```python
from build123d import *

# Parameters (mm, degrees)
ESTRUSIONE_ESTRUSIONE1_DEPTH = 5
SCHIZZO2_R                   = 1.625
TAGLIO_ESTRUSIONE1_DEPTH     = 10.274243706
SCHIZZO3_R                   = 2.5
TAGLIO_ESTRUSIONE2_DEPTH     = 3.5


with BuildPart() as part:
    # Schizzo1 → Estrusione-Estrusione1 (new body, symmetric)
    with BuildSketch(Plane(origin=(0, 0, 0), x_dir=(0, 0, -1), z_dir=(1, 0, 0))):
        Polygon((-21.188457268, 88.94490566), (-26.688457268, 88.94490566), (-26.688457268, 109.666731067), (-40, 122.978273799), (-40, 156.723080253), (-25, 171.723080253), (-25, 168.94490566), (-22.828427125, 168.94490566), (-18.828427125, 172.94490566), (-17.414213562, 171.530692098), (-34.5, 154.44490566), (-34.5, 125.256448392), (-21.188457268, 111.94490566), align=None)
    extrude(amount=ESTRUSIONE_ESTRUSIONE1_DEPTH, both=True)

    # Schizzo2 → Taglio-Estrusione1 (cut, through all)
    with BuildSketch(Plane.XY.offset(26.688457268)):
        with Locations((0, 92.723474812)):
            Circle(SCHIZZO2_R)
    extrude(amount=-TAGLIO_ESTRUSIONE1_DEPTH, mode=Mode.SUBTRACT)

    # Schizzo3 → Taglio-Estrusione2 (cut)
    with BuildSketch(Plane.XY.offset(26.688457268)):
        with Locations((0, 92.723474812)):
            Circle(SCHIZZO3_R)
    extrude(amount=-TAGLIO_ESTRUSIONE2_DEPTH, mode=Mode.SUBTRACT)


solid = part.part
```
Work out the finished part from the listing and answer in its coordinate system (mm). A direction names the side the tool comes from. Coordinates: 2 decimals unless noted, no trailing zeros. Loops run counter-clockwise (first coordinate to the right, second up) from the corner with the lowest first, then second, coordinate; pieces in that order, holes last. Notation, with made-up numbers: (16.25, -35) - (23.25, -35) arc R15 cw to (23.25, -17) - close; hole circle Ø8 at (39.5, 43). An arc over 180 degrees is marked (long way). Use a Markdown table: item, result.
Item 1: For faces 4 (the cylindrical face through (-0.33, 95.2, 24.96)), 5 (the flat face through (0.07, 118.694, 27.937)), 6 (the flat face through (0, 99, 26.688)), 7 (the flat face through (0, 170, 25)), 8 (the flat face through (0, 101, 21.188)), determine the directions among +Z, -Z, +X, -X, +Y, -Y from which every point of the face is accessible in a straight line to the end or side of a thin tool.
Evaluation:
| item | result |
|---|---|
| face 4 | +Z |
| face 5 | -Z, +X, -X |
| face 6 | +Z, +X, -X, -Y |
| face 7 | +X, -X, +Y |
| face 8 | -Z, +X, -X, -Y |
Item 2: Find section A-A, the plane x = 0. Determine the outline of the cut face in (y, z), and give its area (3 significant figures).
Evaluation:
| item | result |
|---|---|
| outline | (88.94, 21.19) - (91.1, 21.19) - (91.1, 23.19) - (90.22, 23.19) - (90.22, 26.69) - (88.94, 26.69) - close; (94.35, 21.19) - (111.94, 21.19) - (125.26, 34.5) - (154.44, 34.5) - (171.53, 17.41) - (172.94, 18.83) - (168.94, 22.83) - (168.94, 25) - (171.72, 25) - (156.72, 40) - (122.98, 40) - (109.67, 26.69) - (95.22, 26.69) - (95.22, 23.19) - (94.35, 23.19) - close |
| area | 490 mm2 |
Item 3: Find section D-D, the plane y = 103. Determine the outline of the cut face in (x, z).
Evaluation:
| item | result |
|---|---|
| outline | (-5, 21.19) - (5, 21.19) - (5, 26.69) - (-5, 26.69) - close |
Item 4: The mould has two halves that part along Z. Classify faces 1 (the flat face through (0, 140, 34.5)), 2 (the flat face through (0.07, 170.917, 20.856)), 3 (the cylindrical face through (0.75, 91.28, 22.2)): +Z half, -Z half, draft (parallel to the pull), parting line (faces both ways), or undercut.
Evaluation:
| item | result |
|---|---|
| face 1 | -Z half |
| face 2 | undercut |
| face 3 | draft |
Item 5: Find section B-B, the plane z = 30.25. Determine the outline of the cut face in (x, y).
Evaluation:
| item | result |
|---|---|
| outline | (-5, 113.23) - (5, 113.23) - (5, 121.01) - (-5, 121.01) - close; (-5, 158.69) - (5, 158.69) - (5, 166.47) - (-5, 166.47) - close |
Item 6: Find section C-C, the plane x = -3.5. Determine the outline of the cut face in (y, z), and give its area (3 significant figures).
Evaluation:
| item | result |
|---|---|
| outline | (88.94, 21.19) - (111.94, 21.19) - (125.26, 34.5) - (154.44, 34.5) - (171.53, 17.41) - (172.94, 18.83) - (168.94, 22.83) - (168.94, 25) - (171.72, 25) - (156.72, 40) - (122.98, 40) - (109.67, 26.69) - (88.94, 26.69) - close |
| area | 514 mm2 |
Item 7: Given pin 1 Ø5 at (x, y) = (2, 138.5) entering from -Z; pin 2 Ø4 at (x, z) = (1.5, 28) entering from +Y; pin 3 Ø1.1 at (x, z) = (0, 23.5) entering from +Y; pin 4 Ø1.9 at (x, y) = (0, 92.72) entering from +Z, each flat-ended and moving along its own axis, determine where each tip first touches the part or whether it passes through.
Evaluation:
| item | result |
|---|---|
| pin 1 | stops at z = 34.5 |
| pin 2 | stops at y = 170.72 |
| pin 3 | stops at y = 168.94 |
| pin 4 | passes through |
Item 8: Consider probe 1 along Y at (x, z) = (0, 22.25); probe 2 along Y at (x, z) = (0, 22.7); probe 3 along Z at (x, y) = (-3.25, 154). Determine where each line is inside the solid, lowest interval first. Write a range as from..to.
Evaluation:
| item | result |
|---|---|
| probe 1 | y = 88.94..91.1, 94.35..113.01, 166.69..169.52 |
| probe 2 | y = 88.94..91.1, 94.35..113.46, 166.24..169.07 |
| probe 3 | z = 34.5..40 |
